The model under review builds one solid part; all positions refer to its coordinate system, in mm. A direction names the side the tool comes from. Round coordinates to 2 decimals unless told otherwise and drop trailing zeros. Order: outer loops, then holes, each group sorted by start corner. A loop starts at its lowest first (then second) coordinate and runs counter-clockwise, first axis right, second up. Notation, with made-up numbers: (-17, 41.25) - (19, 41.25) arc R12 ccw to (19, 58.25) - close; hole circle Ø5 at (-27.75, -33). An arc over 180 degrees is marked (long way). One line per question, with ' | ' between items. Start each with the question number.
Item 1: Add section C-C on y = 149.5. State the section outline as (x, z) points, and give its area (3 significant figures).
Item 2: For L1, parallel to X at y = -16, z = 13.5; L2, parallel to X at y = 38, z = 18.75; L3, parallel to Z at x = -78.5, y = 0, list the stretches that pass through material, from the lowest coordinate up. Write a range as [from, to].
Item 3: Add section A-A on z = 12.5. State the section outline as (x, y) points.
Item 4: Add section B-B on x = 60.5. State the section outline as (y, z) points, and give its area (3 significant figures).
Item 5: Insertion check: pin 1 Ø8 at (x, z) = (-101, 13) entering from +Y; pin 2 Ø8 at (x, y) = (-102.5, -82.5) entering from -Z; pin 3 Ø12.5 at (x, z) = (144, 13) entering from +Y. Each pin has a flat end and moves straight along its axis. Give the tip position at first contact, or say it passes through.
Item 6: Add section D-D on y = 62.5. State the section outline as (x, z) points.
Item 7: Draft analysis for pull direction X (two halves, no side actions). For faces 4 (the face through (-3, 3, 25)), 5 (the face through (200, -76, 12)), 6 (the face through (-150, -55, 12)), state which applies: +X half, -X half, draft (parallel to the pull), parting line (faces both ways), or undercut.
Item 8: Tool access review of faces 1 (the face through (135, -1, 7)), 2 (the face through (1.89, -0.651, 17.457)), 3 (the face through (-200, -74, 12)): name each direction out of +Z, -Z, +X, -X, +Y, -Y from which nothing blocks a thin tool from reaching the whole face with its end or side.
from build123d import *

# Parameters (mm, degrees)
F0_W     = 30
F0_H     = 110
F1_DEPTH = 25
F2_R     = 50
F3_R     = 5
F4_DEPTH = 270


with BuildPart() as f1:
    # F0 (on Top) → F1 (new body)
    with BuildSketch(Plane.XY):
        with BuildLine():
            Line((200, -200), (200, 0))
            ThreePointArc((200, 0), (0, 200), (-200, 0))
            Line((-200, 0), (-200, -200))
            Line((-200, -200), (200, -200))
        make_face()
        with Locations((-150, 0)):
            Rectangle(F0_W, F0_H, mode=Mode.SUBTRACT)
        with Locations((150, 0)):
            Rectangle(F0_W, F0_H, mode=Mode.SUBTRACT)
    extrude(amount=F1_DEPTH)

    # F2
    f2_edges = [f1.edges().sort_by_distance(p)[0] for p in [
        (200, -200, 12.5),
        (-200, -200, 12.5),
    ]]
    fillet(f2_edges, radius=F2_R)

    # F3 (on face) → F4 (cut, through all)
    with BuildSketch(Plane.YZ.offset(135)):
        with Locations((0, 12.5)):
            Circle(F3_R)
    extrude(amount=-F4_DEPTH, mode=Mode.SUBTRACT)


solid = f1.part
Determined:
1) outline: (-132.85, 0) - (132.85, 0) - (132.85, 25) - (-132.85, 25) - close | area: 6,640 mm2
2) L1: [-200, -165], [-135, 135], [165, 200] | L2: [-196.36, -165], [-135, 135], [165, 196.36] | L3: [0, 7.5], [17.5, 25]
3) outline: (-200, -150) arc R50 ccw to (-150, -200) - (150, -200) arc R50 ccw to (200, -150) - (200, 0) arc R200 ccw to (-200, 0) - close; hole (-165, -55) - (-135, -55) - (-135, -5) - (135, -5) - (135, -55) - (165, -55) - (165, 55) - (135, 55) - (135, 5) - (-135, 5) - (-135, 55) - (-165, 55) - close
4) outline: (-200, 0) - (190.63, 0) - (190.63, 25) - (-200, 25) - close; hole circle Ø10 at (0, 12.5) | area: 9,690 mm2
5) pin 1: y = 174.9 | pin 2: z = 0 | pin 3: y = 145
6) outline: (-189.98, 0) - (189.98, 0) - (189.98, 25) - (-189.98, 25) - close
7) face 4: draft | face 5: +X half | face 6: undercut
8) face 1: +Z, -Z | face 2: none | face 3: +Z, -Z, -X, +Y, -Y
